Model file for the job. Use its own axes, mm. Round coordinates to 2 decimals unless told otherwise and drop trailing zeros. Loops run counter-clockwise (first coordinate to the right, second up) from the corner with the lowest first, then second, coordinate; pieces in that order, holes last. Notation, with made-up numbers: (28, 58) -> (61, 58) arc R17 cw to (61, 69) -> close; hole circle Ø1 at (11.25, 76). An arc over 180 degrees is marked (long way). Use a Markdown table: item, result. Add a question column.
```python
from build123d import *

# Parameters (mm, degrees)
CROQUIS1_R              = 35
CROQUIS1_R_2            = 25
SALIENTE_EXTRUIR1_DEPTH = 50
REDONDEO1_R             = 10


with BuildPart() as part:
    # Croquis1 → Saliente-Extruir1 (new body)
    with BuildSketch(Plane(origin=(0, 0, 0), x_dir=(1, 0, 0), z_dir=(0, 1, 0))):
        with BuildLine():
            Line((-147.642857143, 54.949466581), (201.714285714, 39.963248423))
            ThreePointArc((201.714285714, 39.963248423), (240, 0), (201.714285714, -39.963248423))
            Line((201.714285714, -39.963248423), (-147.642857143, -54.949466581))
            ThreePointArc((-147.642857143, -54.949466581), (-205, 0), (-147.642857143, 54.949466581))
        make_face()
        with Locations(Location((-150, 0, 0), (0, 0, 270))):
            Circle(CROQUIS1_R, mode=Mode.SUBTRACT)
        with Locations(Location((200, 0, 0), (0, 0, 270))):
            Circle(CROQUIS1_R_2, mode=Mode.SUBTRACT)
    extrude(amount=SALIENTE_EXTRUIR1_DEPTH)

    # Redondeo1
    redondeo1_edges = [part.edges().sort_by_distance(p)[0] for p in [
        (240, 50, 0),
        (27.035714286, 50, -47.456357502),
        (-205, 50, 0),
        (27.035714286, 0, -47.456357502),
        (240, 0, 0),
        (27.035714286, 0, 47.456357502),
        (-205, 0, 0),
        (27.035714286, 50, 47.456357502),
    ]]
    fillet(redondeo1_edges, radius=REDONDEO1_R)


solid = part.part
```
1) Cut at A-A on z = 0. Write the cut outline in (x, y), and give its area (3 significant figures).
2) Pin check, flat tips, straight feed: pin 1 Ø2 at (x, y) = (-70.5, 29.5) entering from -Z; pin 2 Ø2 at (x, y) = (-19, 9.5) entering from -Z; pin 3 Ø1 at (x, y) = (-14, 6) entering from +Z. Stop position of each tip, or through.
3) Pull direction X, two halves, no side cores. Call faces 1 (the face through (224.787, 24.65, -3.255)), 2 (the face through (29.48, 24.79, 47.35)), 3 (the face through (20, 50, -1)): +X half, -X half, draft (parallel to the pull), parting line (faces both ways), or undercut.
4) Wall check: probe 1 along X at (y, z) = (30, 5); probe 2 along Z at (x, y) = (-151, 31); probe 3 along X at (y, z) = (40.5, -8). Give the ranges that are in metal, low to high. Write a range as from..to.
5) Cut at C-C on y = 46. Write the cut outline in (x, z).
6) Cut at B-B on y = 20. Write the cut outline in (x, z).
Established:
| question | item | result |
|---|---|---|
| 1 | outline | (-205, 10) arc R10 ccw to (-195, 0) -> (-185, 0) -> (-185, 50) -> (-195, 50) arc R10 ccw to (-205, 40) -> close; (-115, 0) -> (175, 0) -> (175, 50) -> (-115, 50) -> close; (225, 0) -> (230, 0) arc R10 ccw to (240, 10) -> (240, 40) arc R10 ccw to (230, 50) -> (225, 50) -> close |
| 1 | area | 16,200 mm^2 |
| 2 | pin 1 | stops at z = -51.68 |
| 2 | pin 2 | stops at z = -49.47 |
| 2 | pin 3 | stops at z = 48.58 |
| 3 | face 1 | undercut |
| 3 | face 2 | +X half |
| 3 | face 3 | draft |
| 4 | probe 1 | x = -204.77..-184.64, -115.36..175.51, 224.49..239.69 |
| 4 | probe 2 | z = -54.99..-34.99, 34.99..54.99 |
| 4 | probe 3 | x = -204.4..-184.07, -115.93..176.31, 223.69..239.18 |
| 5 | outline | (-147.73, -52.95) -> (201.63, -37.97) arc R38 ccw to (201.63, 37.97) -> (-147.73, 52.95) arc R53 ccw (long way) to start; hole circle Ø70 at (-150, 0); hole circle Ø50 at (200, 0) |
| 6 | outline | (-147.64, -54.95) -> (201.71, -39.96) arc R40 ccw to (201.71, 39.96) -> (-147.64, 54.95) arc R55 ccw (long way) to start; hole circle Ø70 at (-150, 0); hole circle Ø50 at (200, 0) |
